```python
from build123d import *


with BuildPart() as part:
    # Sketch → Revolution (revolve)
    with BuildSketch(Plane.XZ):
        Polygon((-2.5, 0), (-5, 0), (-5, -3.5), (-3.5, -5), (-0.75, -5), (-0.5, -6), (-0.5, -7), (0, -7), (0, -3.5), (-2, -3.5), (-2.5, -3), align=None)
    revolve(axis=Axis((0, 0, 0), (0, 0, 1)))


solid = part.part
```
The listing builds one solid part. Answer for the finished solid, in the listing's coordinates (mm). A direction names the side the tool comes from. Give positions to 0.01 mm unless a question says otherwise; leave off trailing zeros. Order: outer loops, then holes, each group sorted by start corner. A loop starts at its lowest first (then second) coordinate and runs counter-clockwise, first axis right, second up.
Item 1: Find the intervals of material crossed by probe 1 along Y at (x, z) = (0, -1.8); probe 2 along Z at (x, y) = (-2.75, -1.25), in increasing order.
From the geometry:
probe 1: y = -5 to -2.5, 2.5 to 5
probe 2: z = -5 to 0
Item 2: Which of the six approach directions +Z, -Z, +X, -X, +Y, -Y give full straight-line access (tool end or side, diameter ignored) to faces 1 (the face through (0, 0, -3.5)), 2 (the face through (2, 2, 0))?
From the geometry:
face 1: +Z
face 2: +Z, +X, -X, +Y, -Y
Item 3: Given pin 1 Ø2 at (x, y) = (1, -0.5) entering from -Z; pin 2 Ø2 at (x, y) = (-0.5, 0) entering from +Z; pin 3 Ø1.5 at (x, z) = (0.5, -6) entering from +Y; pin 4 Ø1.5 at (y, z) = (0, -6) entering from +X, each flat-ended and moving along its own axis, determine where each tip first touches the part or whether it passes through.
From the geometry:
pin 1: stops at z = -7
pin 2: stops at z = -3.5
pin 3: stops at y = 0.65
pin 4: stops at x = 0.69
Item 4: The part is cut by section A-A, the plane x = 0. Give the vertices of the cut face in (y, z).
From the geometry:
outline: (-5, -3.5) - (-3.5, -5) - (-0.75, -5) - (-0.5, -6) - (-0.5, -7) - (0.5, -7) - (0.5, -6) - (0.75, -5) - (3.5, -5) - (5, -3.5) - (5, 0) - (2.5, 0) - (2.5, -3) - (2, -3.5) - (-2, -3.5) - (-2.5, -3) - (-2.5, 0) - (-5, 0) - close
Item 5: The part is cut by section C-C, the plane z = -4.25. Give the vertices of the cut face in (x, y).
From the geometry:
outline: circle Ø8.5 at (0, 0)
Item 6: The part is cut by section D-D, the plane z = -5.5. Give the vertices of the cut face in (x, y) (3 decimals), and give its area (3 significant figures).
From the geometry:
outline: circle Ø1.25 at (0, 0)
area: 1.23 mm2
Item 7: For a pull along Y with two mould halves and no side action, classify faces 3 (the face through (0, -1, -5)), 4 (the face through (0.54, 2.44, -1.48)), 5 (the face through (0.108, 0.488, -6.507)) as pulls with the +Y half, pulls with the -Y half, needs draft (parallel to the pull), parting line crosses it, or undercut.
From the geometry:
face 3: needs draft
face 4: undercut
face 5: parting line crosses it
